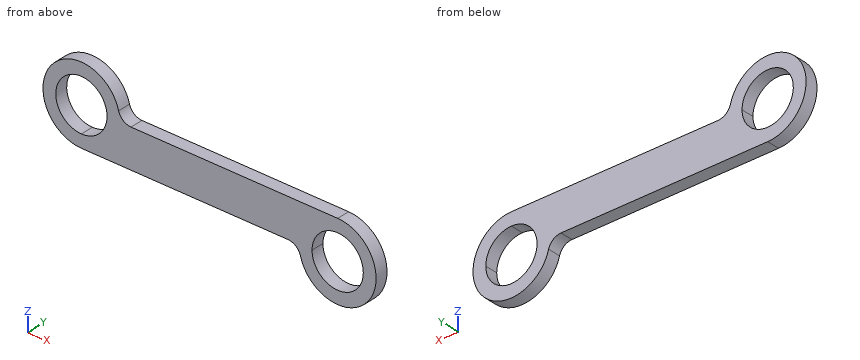
from build123d import *

# Parameters (mm, degrees)
F1_DEPTH = 5
F2_R     = 5


with BuildPart() as f1:
    # F0 (on Front) → F1 (new body)
    with BuildSketch(Plane.XZ):
        with BuildLine():
            Line((-40.3388801531, 15), (-35.3388801531, 15))
            ThreePointArc((-35.3388801531, 15), (-60.9454818709, 25.6066017178), (-50.3388801531, 0))
            Line((-50.3388801531, 0), (-50.3388801531, 5))
            ThreePointArc((-50.3388801531, 5), (-57.409947965, 22.0710678119), (-40.3388801531, 15))
        make_face()
        with BuildLine():
            ThreePointArc((34.6611198469, 0), (39.0545181291, 10.6066017178), (49.6611198469, 15))
            Line((49.6611198469, 15), (-35.3388801531, 15))
            ThreePointArc((-35.3388801531, 15), (-39.7322784353, 4.3933982822), (-50.3388801531, 0))
            Line((-50.3388801531, 0), (34.6611198469, 0))
        make_face()
        with BuildLine():
            ThreePointArc((-50.3388801531, 0), (-39.7322784353, 4.3933982822), (-35.3388801531, 15))
            Line((-35.3388801531, 15), (-40.3388801531, 15))
            ThreePointArc((-40.3388801531, 15), (-43.2678123412, 7.9289321881), (-50.3388801531, 5))
            Line((-50.3388801531, 5), (-50.3388801531, 0))
        make_face()
        with BuildLine():
            ThreePointArc((64.6611198469, 0), (60.2677215647, 10.6066017178), (49.6611198469, 15))
            Line((49.6611198469, 15), (49.6611198469, 10))
            ThreePointArc((49.6611198469, 10), (56.7321876588, 7.0710678119), (59.6611198469, 0))
            ThreePointArc((59.6611198469, 0), (49.6611198469, -10), (39.6611198469, 0))
            Line((39.6611198469, 0), (34.6611198469, 0))
            ThreePointArc((34.6611198469, 0), (49.6611198469, -15), (64.6611198469, 0))
        make_face()
        with BuildLine():
            Line((49.6611198469, 10), (49.6611198469, 15))
            ThreePointArc((49.6611198469, 15), (39.0545181291, 10.6066017178), (34.6611198469, 0))
            Line((34.6611198469, 0), (39.6611198469, 0))
            ThreePointArc((39.6611198469, 0), (42.590052035, 7.0710678119), (49.6611198469, 10))
        make_face()
    extrude(amount=F1_DEPTH)

    # F2
    f2_edges = [f1.edges().sort_by_distance(p)[0] for p in [
        (-35.33888, -2.5, 15),
        (34.66112, -2.5, 0),
    ]]
    fillet(f2_edges, radius=F2_R)


solid = f1.part
Build history of the part. All positions in model axes, mm. Coordinates: 2 decimals unless noted, no trailing zeros. Order: outer loops, then holes, each group sorted by start corner. A loop starts at its lowest first (then second) coordinate and runs counter-clockwise, first axis right, second up. Notation, with made-up numbers: (-18.5, 75) - (-4.5, 75) arc R6 cw to (-4.5, 84) - close; hole circle Ø5 at (-21.75, 11). An arc over 180 degrees is marked (long way). Put each result on its own line as item: value.
1. Probe line 1 along X through (y, z) = (-3.3, 8.5); line 2 along Z through (x, y) = (-17, -2.15); line 3 along X through (y, z) = (-1.5, 16.5). List the from-to ranges inside material, lowest first. Write a range as [from, to].
Answer sheet:
line 1: x = [-63.86, -57.94], [-42.74, 44.39], [54.93, 62.02]
line 2: z = [0, 15]
line 3: x = [-65.26, -60.23], [-40.45, -34.54]
2. Saw through at B-B (x = -45.5). Write the cut outline in (y, z).
Answer sheet:
outline: (-5, 0) - (0, 0) - (0, 6.25) - (-5, 6.25) - close; (-5, 23.75) - (0, 23.75) - (0, 29.2) - (-5, 29.2) - close
3. Saw through at D-D (x = -21.5). Write the cut outline in (y, z).
Answer sheet:
outline: (-5, 0) - (0, 0) - (0, 15) - (-5, 15) - close
4. Drop flat-ended pins along their axis: P1, Ø2.5, axis at x = -28.5, y = -2, coming from the -Z side; P2, Ø10, axis at x = 50.5, z = 15.5, coming from the -Y side; P3, Ø12, axis at x = -50.34, z = 15, coming from the +Y side; P4, Ø1.5, axis at x = 14, y = -2, coming from the +Z side. Give the stop position or say it passes through.
Answer sheet:
P1: stops at z = 0
P2: stops at y = -5
P3: passes through
P4: stops at z = 15
5. Saw through at C-C (z = 16.5). Write the cut outline in (x, y).
Answer sheet:
outline: (-65.26, -5) - (-60.23, -5) - (-60.23, 0) - (-65.26, 0) - close; (-40.45, -5) - (-34.54, -5) - (-34.54, 0) - (-40.45, 0) - close
6. Saw through at A-A (y = -3.8). Write the cut outline in (x, z), and give its area (3 significant figures).
Answer sheet:
outline: (-50.34, 0) - (30.3, 0) arc R5 cw to (35.14, -3.75) arc R15 ccw (long way) to (49.66, 15) - (-30.97, 15) arc R5 cw to (-35.82, 18.75) arc R15 ccw (long way) to start; hole circle Ø20 at (-50.34, 15); hole circle Ø20 at (49.66, 0)
area: 1,940 mm^2
